```python
from build123d import *

# Parameters (mm, degrees)
CYLINDER189_R             = 3.2
CYLINDER189_DEPTH         = 22
CYLINDER190_R             = 3.55
CYLINDER190_DEPTH         = 2
CYLINDER191_R             = 3.55
CYLINDER191_DEPTH         = 1
CYLINDER192_R             = 3.25
CYLINDER192_DEPTH         = 8
CYLINDER193_R             = 4
CYLINDER193_DEPTH         = 5.5
CYLINDER194_R             = 1
CYLINDER194_DEPTH         = 2
FUSION127_PLACEMENT_ANGLE = 180


with BuildPart() as cylinder189:
    # Cylinder189 → Cylinder189 (new body)
    with BuildSketch(Plane.XY.offset(5)):
        Circle(CYLINDER189_R)
    extrude(amount=CYLINDER189_DEPTH)


with BuildPart() as cylinder190:
    # Cylinder190 → Cylinder190 (new body)
    with BuildSketch(Plane.XY.offset(5)):
        Circle(CYLINDER190_R)
    extrude(amount=CYLINDER190_DEPTH)


with BuildPart() as cylinder191:
    # Cylinder191 → Cylinder191 (new body)
    with BuildSketch(Plane.XY.offset(11)):
        Circle(CYLINDER191_R)
    extrude(amount=CYLINDER191_DEPTH)


with BuildPart() as cylinder192:
    # Cylinder192 → Cylinder192 (new body)
    with BuildSketch(Plane.XY.offset(12)):
        Circle(CYLINDER192_R)
    extrude(amount=CYLINDER192_DEPTH)


with BuildPart() as cylinder193:
    # Cylinder193 → Cylinder193 (new body)
    with BuildSketch(Plane.XY.offset(20)):
        Circle(CYLINDER193_R)
    extrude(amount=CYLINDER193_DEPTH)


with BuildPart() as fusion126:
    # Cone001 → Cone001 (revolve)
    with BuildSketch(Plane(origin=(0, 0, 25.5), x_dir=(1, 0, 0), z_dir=(0, -1, 0))):
        Polygon((0, 0), (4, 0), (3.5, 1.5), (0, 1.5), align=None)
    revolve(axis=Axis((0, 0, 25.5), (0, 0, 1)))

    # Fusion126: union Cylinder189, Cylinder190, Cylinder191, Cylinder192, Cylinder193
    add(cylinder189.part)
    add(cylinder190.part)
    add(cylinder191.part)
    add(cylinder192.part)
    add(cylinder193.part)


with BuildPart() as mic001:
    # Cylinder194 → Cylinder194 (new body)
    with BuildSketch(Plane.XY.offset(3)):
        Circle(CYLINDER194_R)
    extrude(amount=CYLINDER194_DEPTH)

    # Fusion127: union Fusion126
    add(fusion126.part)


with BuildPart() as mic001_1:
    # Fusion127 placement: moved
    add(mic001.part.moved(Location((0, -260, -121.25))).rotate(Axis((0, -260, -121.25), (0, 1, 0)), FUSION127_PLACEMENT_ANGLE))


solid = mic001_1.part
```
Geometry check sheet. Reference: the model listing, model coordinates, mm. A direction names the side the tool comes from. Give positions to 0.01 mm unless a question says otherwise; leave off trailing zeros. Loops run counter-clockwise (first coordinate to the right, second up) from the corner with the lowest first, then second, coordinate; pieces in that order, holes last. Notation, with made-up numbers: M -9.5,53.25 L 18.5,53.25 A35 ccw 18.5,88.25 Z; hole C 34.5,55 d4. An arc over 180 degrees is marked long. Write item = value, one per line. Start each with the question number.
1. Section check B-B, the plane x = 0. Enter the section's corners in (y, z).
2. Section check D-D, the plane z = -141.5. Enter the section's corners in (x, y), plus the area to 3 significant figures.
3. Tool access check on faces 1 (the face through (0, -260, -124.25)), 2 (the face through (-1.5, -262.883, -137.194)), 3 (the face through (0.46, -256.48, -132.74)). Record the directions out of +Z, -Z, +X, -X, +Y, -Y that give a thin tool (end or side, any length) a straight path to the whole face; none if there is none.
4. Thickness scan on probe 1 along Z at (x, y) = (-1, -263.25); probe 2 along Z at (x, y) = (1.25, -258); probe 3 along Z at (x, y) = (3, -262.5). Record the ranges inside material, lowest first.
5. Go/stop test with flat-tipped pins: P1, Ø2, axis at x = -3, z = -140, coming from the -Y side; P2, Ø3.5, axis at x = -1.5, y = -259, coming from the +Z side. Record where each tip stops, or that it passes through.
6. Section check C-C, the plane z = -128.75. Enter the section's corners in (x, y).
7. Draft check along Z on faces 4 (the face through (0.694, -263.124, -130.222)), 5 (the face through (2, -257, -141.25)), 6 (the face through (0, -260, -148.25)), 7 (the face through (0.46, -256.48, -127.24)). Enter one of: +Z half, -Z half, draft (parallel to the pull), parting line (faces both ways), or undercut.
8. Section check A-A, the plane y = -260. Enter the section's corners in (x, z).
Values follow:
q1.outline = M -264,-146.75 L -263.5,-148.25 L -256.5,-148.25 L -256,-146.75 L -256,-141.25 L -256.75,-141.25 L -256.75,-133.25 L -256.45,-133.25 L -256.45,-132.25 L -256.8,-132.25 L -256.8,-128.25 L -256.45,-128.25 L -256.45,-126.25 L -259,-126.25 L -259,-124.25 L -261,-124.25 L -261,-126.25 L -263.55,-126.25 L -263.55,-128.25 L -263.2,-128.25 L -263.2,-132.25 L -263.55,-132.25 L -263.55,-133.25 L -263.25,-133.25 L -263.25,-141.25 L -264,-141.25 Z
q2.outline = C 0,-260 d8
q2.area = 50.3 mm^2
q3.face_1 = +Z, +X, -X, +Y, -Y
q3.face_2 = none
q3.face_3 = +Z
q4.probe_1 = -148.25 to -141.25, -133.25 to -132.25, -128.25 to -126.25
q4.probe_2 = -148.25 to -126.25
q4.probe_3 = -147.03 to -141.25
q5.P1 = -262.56
q5.P2 = -124.25
q6.outline = C 0,-260 d6.4
q7.face_4 = undercut
q7.face_5 = undercut
q7.face_6 = -Z half
q7.face_7 = draft
q8.outline = M -4,-146.75 L -3.5,-148.25 L 3.5,-148.25 L 4,-146.75 L 4,-141.25 L 3.25,-141.25 L 3.25,-133.25 L 3.55,-133.25 L 3.55,-132.25 L 3.2,-132.25 L 3.2,-128.25 L 3.55,-128.25 L 3.55,-126.25 L 1,-126.25 L 1,-124.25 L -1,-124.25 L -1,-126.25 L -3.55,-126.25 L -3.55,-128.25 L -3.2,-128.25 L -3.2,-132.25 L -3.55,-132.25 L -3.55,-133.25 L -3.25,-133.25 L -3.25,-141.25 L -4,-141.25 Z
